Design review of the part built by this model. Coordinates are the model's own, in mm. Coordinates: 2 decimals unless noted, no trailing zeros. Write each loop counter-clockwise with the first axis right and the second up, starting at its lowest first coordinate (ties: lowest second). Pieces come first, ordered by that corner, then holes. Notation, with made-up numbers: (53, 75) - (103, 75) arc R17 ccw to (103, 87) - close; hole circle Ø4 at (16.5, 12.5). An arc over 180 degrees is marked (long way). Answer as CSV lines item,"result". Start each with the question number.
Q1. We need section B-B (z = 1.4). Write out the cut boundary in (x, y), plus the area to 3 significant figures.
Q2. We need section A-A (z = 4.5). Write out the cut boundary in (x, y), plus the area to 3 significant figures.
Q3. Clearance check with flat-ended pins moving along their axes: pin 1 (1 mm diameter, centred on x = -26.5, z = 3.5, fed in from -Y); pin 2 (6 mm diameter, centred on x = -28.5, y = 9, fed in from -Z); pin 3 (3 mm diameter, centred on y = 5.5, z = 2, fed in from -X); pin 4 (3 mm diameter, centred on x = -40.5, y = 31.5, fed in from -Z). State where each tip first meets the part, or that it passes through.
Q4. For line 1 along X through (y, z) = (8.5, 1.95); line 2 along Y through (x, z) = (-17, 3.05); line 3 along X through (y, z) = (28.5, 3.15), list the stretches that pass through material, from the lowest coordinate up. Write a range as [from, to].
from build123d import *

# Parameters (mm, degrees)
F1_DEPTH = 5.08
F2_SIZE  = 5.07999


# Not quite as in the source:
# - a fillet or chamfer is up to 0.001 mm smaller than in the source, because OpenCascade refuses the exact size


with BuildPart() as f1:
    # F0 (on Top) → F1 (new body)
    with BuildSketch(Plane.XY):
        with BuildLine():
            Line((0, 0), (0, 44.9222251773))
            ThreePointArc((0, 44.9222251773), (-34.5622433169, 33.8350362208), (-47.7024391294, 0))
            Line((-47.7024391294, 0), (0, 0))
        make_face()
    extrude(amount=F1_DEPTH)

    # F2 (size 5.08 in the source; OpenCascade refuses exactly that, so slightly less here)
    f2_edges = [f1.edges().sort_by_distance(p)[0] for p in [
        (-34.562243, 33.835036, 5.08),
        (-23.85122, 0, 5.08),
    ]]
    chamfer(f2_edges, length=F2_SIZE)


solid = f1.part
Results list:
1,outline,"(-46.38, 1.4) - (0, 1.4) - (0, 43.51) arc R40.76 ccw to start"
1,area,"1,620 mm2"
2,outline,"(-43.29, 4.5) - (0, 4.5) - (0, 40.38) arc R37.66 ccw to start"
2,area,"1,270 mm2"
3,pin 1,"stops at y = 3"
3,pin 2,"stops at z = 0"
3,pin 3,"stops at x = -47.25"
3,pin 4,"passes through"
4,line 1,"x = [-45.51, 0]"
4,line 2,"y = [3.05, 40.57]"
4,line 3,"x = [-35.3, 0]"
